Autodesk Inventor part; units mm, degrees
ref_plane "YZ Plane" through (0, 0, 0) normal (1, 0, 0) x (0, 1, 0)
ref_plane "XZ Plane" through (0, 0, 0) normal (0, 1, 0) x (-1, 0, 0)
ref_plane "XY Plane" through (0, 0, 0) normal (0, 0, 1) x (1, 0, 0)
sketch "Sketch1" plane through (0, 0, 0) normal (0, 0, 1) x (1, 0, 0)
  line L0 (0, 0) -> (-2, 0)
  line L1 (-2, 0) -> (36, 0)
  line L2 (36, 0) -> (36, 17)
  line L3 (36, 17) -> (34, 17)
  line L4 (34, 17) -> (34, 2)
  line L5 (34, 2) -> (0, 2)
  line L6 (0, 2) -> (0, 17)
  line L7 (0, 17) -> (-2, 17)
  line L8 (-2, 17) -> (-2, 0)
  dimension "d8" = 2
  dimension "d9" = 38
  dimension "d10" = 17
  dimension "d11" = 2
  dimension "d12" = 15
extrude "Extrusion1" add sketch "Sketch1" along normal blind 150
sketch "Sketch2" plane through (-2, 17, 150) normal (0, 1, 0) x (1, 0, 0)
  line L0 (0, 150) -> (0, 0)
  line L1 (0, 0) -> (0, 6)
  line L2 (0, 6) -> (2, 6)
  line L3 (2, 150) -> (2, 0)
  line L4 (2, 6) -> (2, 0)
  line L5 (2, 0) -> (0, 0)
  dimension "d13" = 6
  dimension "d14" = 2
extrude "Extrusion2" cut sketch "Sketch2" against normal through all
properties part number "slide1"
The listing builds one solid part. Answer for the finished solid, in the listing's coordinates (mm). A direction names the side the tool comes from. Give positions to 0.01 mm unless a question says otherwise; leave off trailing zeros. Order: outer loops, then holes, each group sorted by start corner. A loop starts at its lowest first (then second) coordinate and runs counter-clockwise, first axis right, second up. Notation, with made-up numbers: (89, -26.5) - (112, -26.5) arc R38 cw to (112, 11.5) - close; hole circle Ø4 at (27, 31). An arc over 180 degrees is marked (long way). Use one line per item in the form item = value. Start each with the question number.
(1) For faces 1 (the flat face through (36, 8, 74)), 2 (the flat face through (0, 9, 71)), determine the directions among +Z, -Z, +X, -X, +Y, -Y from which every point of the face is accessible in a straight line to the end or side of a thin tool.
(2) The mould has two halves that part along X. Classify faces 3 (the flat face through (-2, 9, 71)), 4 (the flat face through (17, 2, 74)), 5 (the flat face through (17, 1, 0)): released by +X, released by -X, zero draft, split by the parting line, or undercut.
(3) A cutting plane is placed at A-A, the plane y = 10.5. Write down the section's boundary in (x, z), then the cut area to 3 significant figures.
(4) A cutting plane is placed at C-C, the plane x = 9.5. Write down the section's boundary in (y, z).
(5) Consider line 1 (X direction, y = 14, z = 135.5); line 2 (Y direction, x = 4, z = 97). Determine where each line is inside the solid, lowest interval first. Write a range as from..to.
(6) A cutting plane is placed at B-B, the plane z = 128. Write down the section's boundary in (x, y), then the cut area to 3 significant figures.
(7) Flat-ended cylindrical pins translate along their axes: pin 1 Ø1.6 at (y, z) = (1, 146) entering from -X; pin 2 Ø2 at (x, y) = (20, 2.5) entering from +Z; pin 3 Ø2 at (x, y) = (-1, 10) entering from +Z. Find the tip coordinate at first contact, or state that the pin passes through.
Ans:
q1.face_1 = +Z, -Z, +X, +Y, -Y
q1.face_2 = +Z, -Z, +Y
q2.face_3 = released by -X
q2.face_4 = undercut
q2.face_5 = zero draft
q3.outline = (-2, 0) - (0, 0) - (0, 144) - (-2, 144) - close; (34, 0) - (36, 0) - (36, 150) - (34, 150) - close
q3.area = 588 mm^2
q4.outline = (0, 0) - (2, 0) - (2, 150) - (0, 150) - close
q5.line_1 = -2..0, 34..36
q5.line_2 = 0..2
q6.outline = (-2, 0) - (36, 0) - (36, 17) - (34, 17) - (34, 2) - (0, 2) - (0, 17) - (-2, 17) - close
q6.area = 136 mm^2
q7.pin_1 = 0
q7.pin_2 = 150
q7.pin_3 = 144
